Part print with two shaded views. Sizes in mm from the minimum x, y, z corner. A direction names the side the tool comes from. Coordinates: 2 decimals unless noted, no trailing zeros. Loops run counter-clockwise (first coordinate to the right, second up) from the corner with the lowest first, then second, coordinate; pieces in that order, holes last. Notation, with made-up numbers: (8.25, 53.5) -> (31.25, 53.5) arc R21 ccw to (31.25, 62.5) -> close; hole circle Ø7 at (-30.75, -31). An arc over 180 degrees is marked (long way). Return JSON: item names as keys, results as strings. Group by question number.
(1) Mould opens along X. For the marked faces 1, 2 and 3 say: pulls with the +X half, pulls with the -X half, needs draft (parallel to the pull), parting line crosses it, or undercut.
(2) Flat gauge pins, fed straight in: pin 1 Ø5.5 at (x, y) = (72, 7.5) entering from +Z (1 decimal); pin 2 Ø1 at (y, z) = (10, 67) entering from +X; pin 3 Ø4.5 at (x, y) = (33.5, 11) entering from +Z. Where does each tip first touch, or does it go through?
(3) Saw through at A-A on x = 58. Write the cut outline in (y, z), then the cut area to 3 significant figures.
(4) Saw through at C-C on y = 9.5. Write the cut outline in (x, z), then the cut area to 3 significant figures.
(5) Saw through at D-D on z = 59.5. Write the cut outline in (x, y), then the cut area to 3 significant figures.
(6) Probe L1, parallel to X at y = 7.25, z = 31.5; L2, parallel to Z at x = 53, y = 11.5 (1 decimal); L3, parallel to Z at x = 56, y = 5.25. List the from-to ranges inside material, lowest first.
(7) Tool access for the marked faces 4, 5 and 6: list every direction of +Z, -Z, +X, -X, +Y, -Y with a clear straight run to the whole face (end or side of a thin tool).
(8) Saw through at B-B on z = 81.5. Write the cut outline in (x, y).
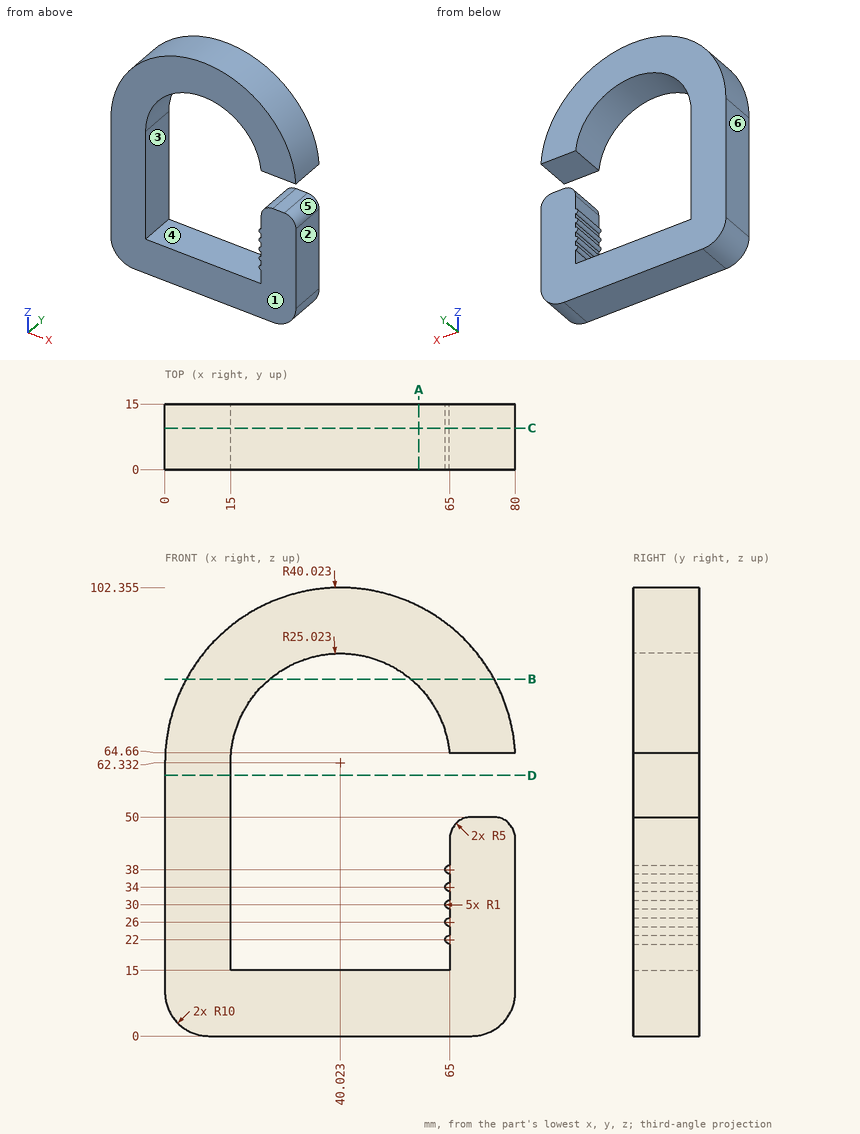
Geometry results:
{
 "1": {"face 1": "needs draft", "face 2": "pulls with the +X half", "face 3": "undercut"},
 "2": {"pin 1": "z = 89.7", "pin 2": "x = 79.83", "pin 3": "z = 102.13"},
 "3": {"outline": "(0, 0) -> (15, 0) -> (15, 15) -> (0, 15) -> close; (0, 79.74) -> (15, 79.74) -> (15, 98.09) -> (0, 98.09) -> close", "area": "500 mm²"},
 "4": {"outline": "(0, 10) arc R10 ccw to (10, 0) -> (70, 0) arc R10 ccw to (80, 10) -> (80, 45) arc R5 ccw to (75, 50) -> (70, 50) arc R5 ccw to (65, 45) -> (65, 39) arc R1 ccw to (65, 37) -> (65, 35) arc R1 ccw to (65, 33) -> (65, 31) arc R1 ccw to (65, 29) -> (65, 27) arc R1 ccw to (65, 25) -> (65, 23) arc R1 ccw to (65, 21) -> (65, 15) -> (15, 15) -> (15, 62.33) arc R25.02 cw to (64.94, 64.66) -> (79.98, 64.66) arc R40.02 ccw to (0, 62.33) -> close", "area": "3,890 mm²"},
 "5": {"outline": "(0, 0) -> (15, 0) -> (15, 15) -> (0, 15) -> close", "area": "225 mm²"},
 "6": {"L1": "0 to 15, 65 to 80", "L2": "0 to 15, 83.7 to 100.2", "L3": "0 to 15, 81.59 to 99.03"},
 "7": {"face 4": "+Y, -Y", "face 5": "+X, +Y, -Y", "face 6": "+Z, -Z, -X, +Y, -Y"},
 "8": {"outline": "(4.89, 0) -> (23.94, 0) -> (23.94, 15) -> (4.89, 15) -> close; (56.11, 0) -> (75.16, 0) -> (75.16, 15) -> (56.11, 15) -> close"}
}
